Check sheet for the modelled part. Datum: model origin and axes. Units: mm. Give positions to 0.01 mm unless a question says otherwise; leave off trailing zeros. Loops run counter-clockwise (first coordinate to the right, second up) from the corner with the lowest first, then second, coordinate; pieces in that order, holes last. Notation, with made-up numbers: (63.5, 57.25) -> (120.5, 57.25) arc R22 cw to (120.5, 80.25) -> close; hole circle Ø6 at (8.5, 88.5). An arc over 180 degrees is marked (long way). Answer as CSV lines item,"result". Start each with the question number.
(1) Section check B-B on z = 2. Enter the section's corners in (x, y).
(2) Material ranges on line 1 (X direction, y = 3.5, z = 5.75); line 2 (X direction, y = 8, z = 4.75); line 3 (Z direction, x = 13, y = 1), recorded low to high. Write a range as from..to.
(3) Section check A-A on x = 4.75. Enter the section's corners in (y, z).
(4) Release check for a two-part mould opening along X. For faces 1 (the face through (0.285, 5.324, 7.699)), 2 (the face through (18.499, 5.324, 7.715)), 3 (the face through (0.28, 5.324, 0.674)) record: pulls with the +X half, pulls with the -X half, needs draft (parallel to the pull), parting line crosses it, or undercut.
(5) Gauge pin test, flat end, axial feed: pin 1 Ø2.5 at (x, z) = (4.35, 5.78) entering from -Y. Record the tip position at first contact, or that the pin passes through.
(6) Section check C-C on y = 5. Enter the section's corners in (x, z).
(7) Section check D-D on z = 6. Enter the section's corners in (x, y).
from build123d import *

# Parameters (mm, degrees)
EXTRUDE_1_DEPTH   = 10.5
FILLET_1_R        = 1
HOLE_WIZARD_M31_D = 3.4
FILLET_2_R        = 0.5


with BuildPart() as part:
    # Эскиз1 → Бобышка-Вытянуть1 (new body)
    with BuildSketch(Plane(origin=(0, 0, 0), x_dir=(1, 0, 0), z_dir=(0, 1, 0))):
        with BuildLine():
            Line((0, 0), (0, -8))
            Line((0, -8), (18.8, -8))
            Line((18.8, -8), (18.8, 0))
            ThreePointArc((18.8, 0), (9.4, -3.835773145), (0, 0))
        make_face()
    extrude(amount=EXTRUDE_1_DEPTH)

    # Скругление1
    fillet_1_edges = [part.edges().sort_by_distance(p)[0] for p in [
        (18.8, 5.25, 8),
        (0, 5.25, 8),
    ]]
    fillet(fillet_1_edges, radius=FILLET_1_R)

    # Отверстие с зазором M31 (through all)
    with Locations(Plane(origin=(0, 10.5, 0), x_dir=(1, 0, 0), z_dir=(0, 1, 0))):
        with Locations((4.350247301, -5.779226371), (14.350247301, -5.779226371)):
            Hole(HOLE_WIZARD_M31_D / 2)

    # Скругление2
    fillet_2_edges = [part.edges().sort_by_distance(p)[0] for p in [
        (18.8, 5.25, 0),
        (0, 5.25, 0),
    ]]
    fillet(fillet_2_edges, radius=FILLET_2_R)


solid = part.part
Working result:
1,outline,"(0, 0) -> (2.62, 0) -> (2.62, 10.5) -> (0, 10.5) -> close; (16.18, 0) -> (18.8, 0) -> (18.8, 10.5) -> (16.18, 10.5) -> close"
2,line 1,"x = 0..2.65, 6.05..12.65, 16.05..18.8"
2,line 2,"x = 0..3, 5.7..13, 15.7..18.8"
2,line 3,"z = 3.34..4.75, 6.81..8"
3,outline,"(0, 3.01) -> (10.5, 3.01) -> (10.5, 4.13) -> (0, 4.13) -> close; (0, 7.43) -> (10.5, 7.43) -> (10.5, 8) -> (0, 8) -> close"
4,face 1,"pulls with the -X half"
4,face 2,"pulls with the +X half"
4,face 3,"undercut"
5,pin 1,"passes through"
6,outline,"(0, 1.12) arc R0.5 ccw to (0.82, 0.74) arc R13.44 cw to (17.98, 0.74) arc R0.5 ccw to (18.8, 1.12) -> (18.8, 7) arc R1 ccw to (17.8, 8) -> (1, 8) arc R1 ccw to (0, 7) -> close; hole circle Ø3.4 at (4.35, 5.78); hole circle Ø3.4 at (14.35, 5.78)"
7,outline,"(0, 0) -> (2.66, 0) -> (2.66, 10.5) -> (0, 10.5) -> close; (6.04, 0) -> (12.66, 0) -> (12.66, 10.5) -> (6.04, 10.5) -> close; (16.04, 0) -> (18.8, 0) -> (18.8, 10.5) -> (16.04, 10.5) -> close"
